Geometry: final body of the model. Coordinates: model frame, mm. A direction names the side the tool comes from. Coordinates: 2 decimals unless noted, no trailing zeros. Loops run counter-clockwise (first coordinate to the right, second up) from the corner with the lowest first, then second, coordinate; pieces in that order, holes last. Notation, with made-up numbers: (86, 39.25) -> (114, 39.25) arc R15 cw to (114, 60.25) -> close; hole circle Ø6 at (-26, 7). An arc over 180 degrees is marked (long way). One line per item, written item: value. Start each with the question number.
Item 1: Section query D-D on z = -9. Return loops of the section in (x, y), then the cut area to 3 significant figures.
Item 2: Ray query, probe 1 along Z at (x, y) = (2.25, -7.5); probe 2 along Y at (x, z) = (10, -0.05); probe 3 along Z at (x, y) = (4, 19.5). Return the intervals inside material, ascending. Write a range as from..to.
Item 3: Mould query, pull axis Y, two halves, no side actions, for faces 5 (the cylindrical face through (1.48, -21.75, -20.04)), 6 (the cylindrical face through (2, 24, -23)), 7 (the flat face through (7, 0, 1.5)). Classes: +Y half, -Y half, draft (parallel to the pull), parting line (faces both ways), or undercut.
Item 4: Section query C-C on y = -16. Return loops of the section in (x, z), then the cut area to 3 significant figures.
Item 5: Contact query for flat-ended pins moving along their axis: pin 1 Ø6 at (y, z) = (8.5, -12) entering from +X; pin 2 Ø1.5 at (y, z) = (-12, 15) entering from -X; pin 3 Ø0.9 at (x, z) = (6, 0) entering from +Y; pin 4 Ø8 at (x, y) = (10, 18) entering from +Z. Output: stop coordinate, or through.
Item 6: Section query B-B on y = 0. Return loops of the section in (x, z), then the cut area to 3 significant figures.
Item 7: Set-up query: faces 1 (the flat face through (7, 18, 1.5)), 2 (the flat face through (1, 0, -8.25)), 3 (the flat face through (7, 0, -1.5)), 4 (the flat face through (7, 4, 0)). Return all of +Z, -Z, +X, -X, +Y, -Y with unobstructed straight access to the full face (end or side cutting, diameter ignored); none if empty.
Item 8: Section query A-A on z = 10. Return loops of the section in (x, y).
from build123d import *

# Parameters (mm, degrees)
SKETCH_1_W      = 50
SKETCH_1_H      = 50
SKETCH_1_R      = 1.75
EXTRUDE_1_DEPTH = 3
SKETCH_2_R      = 4
SKETCH_2_R_2    = 2.5
EXTRUDE_2_DEPTH = 1.5
FILLET_1_R      = 5


with BuildPart() as part:
    # 草图1 → 凸台-拉伸1 (new body)
    # profile 1 of 4: a face of its own
    with BuildSketch(Plane(origin=(0, 0, 0), x_dir=(0, 0, -1), z_dir=(1, 0, 0))):
        Rectangle(SKETCH_1_W, SKETCH_1_H)
        with BuildLine():
            Line((-21.75, -20), (-21.75, 20))
            ThreePointArc((-21.75, 20), (-20, 21.75), (-18.25, 20))
            Line((-18.25, 20), (-18.25, -20))
            ThreePointArc((-18.25, -20), (-20, -21.75), (-21.75, -20))
        make_face(mode=Mode.SUBTRACT)
        with BuildLine():
            Line((-11.75, -20), (-11.75, 20))
            ThreePointArc((-11.75, 20), (-10, 21.75), (-8.25, 20))
            Line((-8.25, 20), (-8.25, -20))
            ThreePointArc((-8.25, -20), (-10, -21.75), (-11.75, -20))
        make_face(mode=Mode.SUBTRACT)
        with BuildLine():
            Line((-1.75, -20), (-1.75, 20))
            ThreePointArc((-1.75, 20), (0, 21.75), (1.75, 20))
            Line((1.75, 20), (1.75, -20))
            ThreePointArc((1.75, -20), (0, -21.75), (-1.75, -20))
        make_face(mode=Mode.SUBTRACT)
        with BuildLine():
            Line((8.25, -20), (8.25, 20))
            ThreePointArc((8.25, 20), (10, 21.75), (11.75, 20))
            Line((11.75, 20), (11.75, -20))
            ThreePointArc((11.75, -20), (10, -21.75), (8.25, -20))
        make_face(mode=Mode.SUBTRACT)
        with BuildLine():
            Line((18.25, -20), (18.25, 20))
            ThreePointArc((18.25, 20), (20, 21.75), (21.75, 20))
            Line((21.75, 20), (21.75, -20))
            ThreePointArc((21.75, -20), (20, -21.75), (18.25, -20))
        make_face(mode=Mode.SUBTRACT)
    # profile 2 of 4: a face of its own
    with BuildSketch(Plane(origin=(0, 0, 0), x_dir=(0, 0, -1), z_dir=(1, 0, 0))):
        with BuildLine():
            ThreePointArc((1.75, 20), (0, 18.25), (-1.75, 20))
            Line((-1.75, 20), (-1.75, -20))
            ThreePointArc((-1.75, -20), (0, -18.25), (1.75, -20))
            Line((1.75, -20), (1.75, 20))
        make_face()
    # profile 3 of 4: a face of its own
    with BuildSketch(Plane(origin=(0, 0, 0), x_dir=(0, 0, -1), z_dir=(1, 0, 0))):
        with Locations((0, 20)):
            Circle(SKETCH_1_R)
    # profile 4 of 4: a face of its own
    with BuildSketch(Plane(origin=(0, 0, 0), x_dir=(0, 0, -1), z_dir=(1, 0, 0))):
        with Locations((0, -20)):
            Circle(SKETCH_1_R)
    extrude(amount=EXTRUDE_1_DEPTH)

    # 草图2 → 凸台-拉伸2 (add, symmetric)
    # profile 1 of 4: a face of its own
    with BuildSketch(Plane.XY):
        with BuildLine():
            Line((0, 14), (10, 14))
            ThreePointArc((10, 14), (6, 18), (10, 22))
            Line((10, 22), (0, 22))
            Line((0, 22), (0, 14))
        make_face()
    # profile 2 of 4: a face of its own
    with BuildSketch(Plane.XY):
        with Locations((10, 18)):
            Circle(SKETCH_2_R)
        with Locations((10, 18)):
            Circle(SKETCH_2_R_2, mode=Mode.SUBTRACT)
    # profile 3 of 4: a face of its own
    with BuildSketch(Plane.XY):
        with Locations((10, 0)):
            Circle(SKETCH_2_R)
        with Locations((10, 0)):
            Circle(SKETCH_2_R_2, mode=Mode.SUBTRACT)
    # profile 4 of 4: a face of its own
    with BuildSketch(Plane.XY):
        with BuildLine():
            Line((0, -4), (10, -4))
            ThreePointArc((10, -4), (6, 0), (10, 4))
            Line((10, 4), (0, 4))
            Line((0, 4), (0, -4))
        make_face()
    extrude(amount=EXTRUDE_2_DEPTH, both=True)

    # 圆角1
    fillet_1_edges = [part.edges().sort_by_distance(p)[0] for p in [
        (1.5, -25, -25),
        (1.5, -25, 25),
        (1.5, 25, 25),
        (1.5, 25, -25),
    ]]
    fillet(fillet_1_edges, radius=FILLET_1_R)


solid = part.part
Reply:
1. outline: (0, -25) -> (3, -25) -> (3, -21.44) -> (0, -21.44) -> close; (0, 21.44) -> (3, 21.44) -> (3, 25) -> (0, 25) -> close
1. area: 21.4 mm²
2. probe 1: z = -25..-21.75, -18.25..-11.75, -8.25..8.25, 11.75..18.25, 21.75..25
2. probe 2: y = -4..-2.5, 2.5..4, 14..15.5, 20.5..22
2. probe 3: z = -1.5..1.5
3. face 5: undercut
3. face 6: +Y half
3. face 7: draft
4. outline: (0, -25) -> (3, -25) -> (3, -21.75) -> (0, -21.75) -> close; (0, -18.25) -> (3, -18.25) -> (3, -11.75) -> (0, -11.75) -> close; (0, -8.25) -> (3, -8.25) -> (3, 8.25) -> (0, 8.25) -> close; (0, 11.75) -> (3, 11.75) -> (3, 18.25) -> (0, 18.25) -> close; (0, 21.75) -> (3, 21.75) -> (3, 25) -> (0, 25) -> close
4. area: 108 mm²
5. pin 1: stops at x = 3
5. pin 2: stops at x = 0
5. pin 3: stops at y = 22
5. pin 4: stops at z = 1.5
6. outline: (0, -25) -> (3, -25) -> (3, -21.75) -> (0, -21.75) -> close; (0, -18.25) -> (3, -18.25) -> (3, -11.75) -> (0, -11.75) -> close; (0, -8.25) -> (3, -8.25) -> (3, -1.5) -> (7.5, -1.5) -> (7.5, 1.5) -> (3, 1.5) -> (3, 8.25) -> (0, 8.25) -> close; (0, 11.75) -> (3, 11.75) -> (3, 18.25) -> (0, 18.25) -> close; (0, 21.75) -> (3, 21.75) -> (3, 25) -> (0, 25) -> close; (12.5, -1.5) -> (14, -1.5) -> (14, 1.5) -> (12.5, 1.5) -> close
6. area: 126 mm²
7. face 1: +Z, +X, +Y, -Y
7. face 2: +X, -X
7. face 3: -Z, +X, +Y, -Y
7. face 4: +Z, -Z, +X
8. outline: (0, -25) -> (3, -25) -> (3, -21.75) -> (0, -21.75) -> close; (0, 21.75) -> (3, 21.75) -> (3, 25) -> (0, 25) -> close
